Model file for the job. Use its own axes, mm. A direction names the side the tool comes from. Round coordinates to 2 decimals unless told otherwise and drop trailing zeros. Order: outer loops, then holes, each group sorted by start corner. A loop starts at its lowest first (then second) coordinate and runs counter-clockwise, first axis right, second up. Notation, with made-up numbers: (72, 79.25) - (82, 79.25) arc R25 cw to (82, 108.25) - close; hole circle Ø5 at (6.5, 74.5). An arc over 180 degrees is marked (long way). Put each result on its own line as item: value. Start each with the question number.
Item 1: Pin check, flat tips, straight feed: pin 1 Ø1.5 at (y, z) = (192, -2) entering from -X; pin 2 Ø3 at (x, z) = (-2, -4) entering from +Y; pin 3 Ø1.5 at (y, z) = (194, -5.5) entering from +X. Stop position of each tip, or through.
Item 2: Saw through at A-A on y = 213.5. List the corners of the cut face in (x, z).
Item 3: Which spindle directions (+Z, -Z, +X, -X, +Y, -Y) get a long thin tool onto all of the face, cutting with end or side? Do faces 1 (the face through (62, 252.601, -3)), 2 (the face through (0, 187.601, -3)), 3 (the face through (75, 127.601, -3)). Say none if no direction does.
Item 4: Saw through at B-B on x = -35. List the corners of the cut face in (y, z), plus the area to 3 significant figures.
Item 5: Probe probe 1 along Y at (x, z) = (2, -2); probe 2 along Y at (x, z) = (-24.5, -5); probe 3 along Y at (x, z) = (18, -5.75). List the from-to ranges inside material, lowest first.
```python
from build123d import *

# Parameters (mm, degrees)
SKETCH1_R           = 19.125454448
SKETCH1_W           = 20
SKETCH1_H           = 1.5875
SKETCH1_W_2         = 6.35
SKETCH1_H_2         = 20
SKETCH1_H_3         = 6.35
SKETCH1_R_2         = 6.35
BOSS_EXTRUDE1_DEPTH = 6.35


with BuildPart() as part:
    # Sketch1 → Boss-Extrude1 (new body)
    with BuildSketch(Plane.XY):
        Polygon((71.384937154, 207.60103085), (71.384937154, 227.60103085), (71.384937154, 252.60103085), (52.734937154, 252.60103085), (32.734937154, 252.60103085), (2.734937154, 252.60103085), (2.734937154, 227.60103085), (2.734937154, 207.60103085), (2.734937154, 187.60103085), (2.734937154, 167.60103085), (2.734937154, 147.60103085), (2.734937154, 127.60103085), (2.734937154, 102.60103085), (2.734937154, 101.01353085), (-24.765062846, 101.01353085), (-44.765062846, 101.01353085), (-65.915062846, 101.01353085), (-65.915062846, 81.01353085), (-65.915062846, 61.01353085), (-65.915062846, 41.01353085), (-65.915062846, 21.01353085), (-65.915062846, 1.01353085), (-47.265062846, 1.01353085), (-27.265062846, 1.01353085), (-7.265062846, 1.01353085), (12.734937154, 1.01353085), (32.734937154, 1.01353085), (52.734937154, 1.01353085), (71.384937154, 1.01353085), (71.384937154, 21.01353085), (71.384937154, 41.01353085), (71.384937154, 61.01353085), (71.384937154, 81.01353085), (71.384937154, 127.60103085), (71.384937154, 147.60103085), (71.384937154, 167.60103085), (71.384937154, 187.60103085), align=None)
        with Locations((42.734937154, 31.01353085)):
            Circle(SKETCH1_R, mode=Mode.SUBTRACT)
        with Locations((-34.765062846, 101.80728085)):
            Rectangle(SKETCH1_W, SKETCH1_H)
        with Locations((-69.090062846, 71.01353085)):
            Rectangle(SKETCH1_W_2, SKETCH1_H_2)
        with Locations((-69.090062846, 31.01353085)):
            Rectangle(SKETCH1_W_2, SKETCH1_H_2)
        with Locations((-37.265062846, -2.16146915)):
            Rectangle(SKETCH1_W, SKETCH1_H_3)
        with Locations((2.734937154, -2.16146915)):
            Rectangle(SKETCH1_W, SKETCH1_H_3)
        with Locations((42.734937154, -2.16146915)):
            Rectangle(SKETCH1_W, SKETCH1_H_3)
        with Locations((74.559937154, 31.01353085)):
            Rectangle(SKETCH1_W_2, SKETCH1_H_2)
        with Locations((74.559937154, 71.01353085)):
            Rectangle(SKETCH1_W_2, SKETCH1_H_2)
        with Locations((74.559937154, 137.60103085)):
            Rectangle(SKETCH1_W_2, SKETCH1_H_2)
        with Locations((74.559937154, 177.60103085)):
            Rectangle(SKETCH1_W_2, SKETCH1_H_2)
        with Locations((74.559937154, 217.60103085)):
            Rectangle(SKETCH1_W_2, SKETCH1_H_2)
        with Locations((42.734937154, 255.77603085)):
            Rectangle(SKETCH1_W, SKETCH1_H_3)
        with Locations((-0.440062846, 217.60103085)):
            Rectangle(SKETCH1_W_2, SKETCH1_H_2)
        with Locations((-0.440062846, 177.60103085)):
            Rectangle(SKETCH1_W_2, SKETCH1_H_2)
        with Locations((-0.440062846, 137.60103085)):
            Rectangle(SKETCH1_W_2, SKETCH1_H_2)
        with Locations((42.734937154, 31.01353085)):
            Circle(SKETCH1_R)
        with Locations((42.734937154, 31.01353085)):
            Circle(SKETCH1_R_2, mode=Mode.SUBTRACT)
    extrude(amount=-BOSS_EXTRUDE1_DEPTH)


solid = part.part
```
Results found:
1. pin 1: stops at x = 2.73
1. pin 2: stops at y = 227.6
1. pin 3: stops at x = 71.38
2. outline: (-3.62, -6.35) - (77.73, -6.35) - (77.73, 0) - (-3.62, 0) - close
3. face 1: +Z, -Z, +X, +Y
3. face 2: +Z, -Z, -X
3. face 3: +Z, -Z, +X
4. outline: (-5.34, -6.35) - (102.6, -6.35) - (102.6, 0) - (-5.34, 0) - close
4. area: 685 mm²
5. probe 1: y = -5.34 to 101.01, 127.6 to 147.6, 167.6 to 187.6, 207.6 to 227.6
5. probe 2: y = 1.01 to 101.01
5. probe 3: y = 1.01 to 252.6
